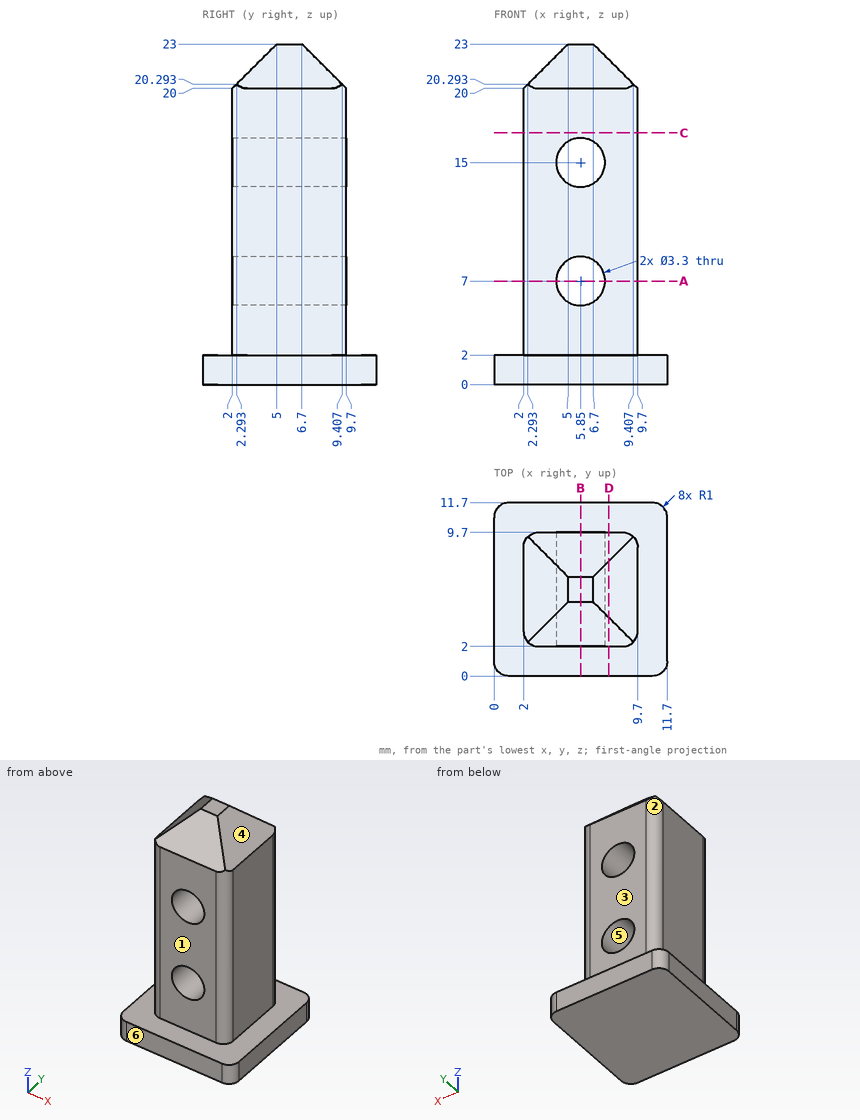
Source: three-view drawing plus pictorial views. Frame: mm from the lowest corner of the part. A direction names the side the tool comes from. Give positions to 0.01 mm unless a question says otherwise; leave off trailing zeros. Write each loop counter-clockwise with the first axis right and the second up, starting at its lowest first coordinate (ties: lowest second). Pieces come first, ordered by that corner, then holes.
(1) Mould query, pull axis Z, two halves, no side actions, for the marked faces 4, 5 and 6. Classes: released by +Z, released by -Z, zero draft, split by the parting line, or undercut.
(2) Cut plane C-C, the plane z = 17. Return loops of the section in (x, y), then the cut area to 3 significant figures.
(3) Cut plane A-A, the plane z = 7. Return loops of the section in (x, y).
(4) Ray query, line 1 (Z direction, x = 5.85, y = 6.25); line 2 (Z direction, x = 5.25, y = 8.75); line 3 (X direction, y = 4, z = 10.5). Return the intervals inside material, ascending.
(5) Cut plane D-D, the plane x = 7.75. Return loops of the section in (y, z), then the cut area to 3 significant figures.
(6) Access query for the marked faces 1, 2 and 3. Directions: +Z, -Z, +X, -X, +Y, -Y. A direction counts if a zero-diameter tool reaches every point of the face in a straight line with its end or side. Return the directions, or none.
(7) Cut plane B-B, the plane x = 5.85. Return loops of the section in (y, z).
(8) First-contact query: P1, Ø2.5, axis at x = 5.85, z = 15, coming from the -Y side; P2, Ø6.5, axis at x = 4.5, z = 10.5, coming from the +Y side; P3, Ø6, axis at y = 4.5, z = 17, coming from the +X side; P4, Ø3, axis at y = 10.5, z = 12, coming from the -X side. Flat tips, straight axial feed; report the tip coordinate or a pass-through.
Values follow:
1. face 4: released by +Z
1. face 5: undercut
1. face 6: zero draft
2. outline: (2, 3) arc R1 ccw to (3, 2) - (8.7, 2) arc R1 ccw to (9.7, 3) - (9.7, 8.7) arc R1 ccw to (8.7, 9.7) - (3, 9.7) arc R1 ccw to (2, 8.7) - close
2. area: 58.4 mm2
3. outline: (2, 3) arc R1 ccw to (3, 2) - (4.2, 2) - (4.2, 9.7) - (3, 9.7) arc R1 ccw to (2, 8.7) - close; (7.5, 2) - (8.7, 2) arc R1 ccw to (9.7, 3) - (9.7, 8.7) arc R1 ccw to (8.7, 9.7) - (7.5, 9.7) - close
4. line 1: z = 0 to 5.35, 8.65 to 13.35, 16.65 to 23
4. line 2: z = 0 to 5.46, 8.54 to 13.46, 16.54 to 20.95
4. line 3: x = 2 to 9.7
5. outline: (0, 0) - (11.7, 0) - (11.7, 2) - (9.7, 2) - (9.7, 20) - (7.75, 21.95) - (3.95, 21.95) - (2, 20) - (2, 2) - (0, 2) - close
5. area: 173 mm2
6. face 1: +Z, +X, -X, -Y
6. face 2: +Z, -X, +Y
6. face 3: +Z, +X, -X, +Y
7. outline: (0, 0) - (11.7, 0) - (11.7, 2) - (9.7, 2) - (9.7, 5.35) - (2, 5.35) - (2, 2) - (0, 2) - close; (2, 8.65) - (9.7, 8.65) - (9.7, 13.35) - (2, 13.35) - close; (2, 16.65) - (9.7, 16.65) - (9.7, 20) - (6.7, 23) - (5, 23) - (2, 20) - close
8. P1: passes through
8. P2: stops at y = 9.7
8. P3: stops at x = 9.7
8. P4: stops at x = 2.05
